For this review, take the finished solid that the model builds, in its own axes (mm). A direction names the side the tool comes from. Coordinates: 2 decimals unless noted, no trailing zeros. Write each loop counter-clockwise with the first axis right and the second up, starting at its lowest first coordinate (ties: lowest second). Pieces come first, ordered by that corner, then holes. Notation, with made-up numbers: (-32, -35) - (8, -35) arc R30 ccw to (8, -4) - close; hole circle Ø1 at (28.25, 20.5). An arc over 180 degrees is marked (long way). Write each question's results on one line, items separated by ' | '.
from build123d import *

# Parameters (mm, degrees)
F0_R     = 12.7
F1_DEPTH = 73.66
F2_R     = 5.1125641025
F3_DEPTH = 73.661
F3_TAPER = -2.9356734464
F4_R     = 12.7
F5_DEPTH = 15.24
F8_D     = 20.447
F8_DEPTH = 19.7358
F8_TIP   = 6.1428985386


with BuildPart() as f1:
    # F0 (on Top) → F1 (new body)
    with BuildSketch(Plane.XY):
        Circle(F0_R)
    extrude(amount=F1_DEPTH)

    # F2 (on Top) → F3 (cut, through all)
    with BuildSketch(Plane.XY):
        Circle(F2_R)
    extrude(amount=F3_DEPTH, taper=F3_TAPER, mode=Mode.SUBTRACT)

    # F4 (on face) → F5 (join)
    with BuildSketch(Plane.XY.offset(73.66)):
        Circle(F4_R)
    extrude(amount=F5_DEPTH)

    # F8
    with Locations(Plane.XY.offset(88.9)):
        with Locations((0, 0)):
            Hole(F8_D / 2, depth=F8_DEPTH)
            with Locations((0, 0, -(F8_DEPTH + F8_TIP / 2))):  # 118° drill point
                Cone(0, F8_D / 2, F8_TIP, mode=Mode.SUBTRACT)


solid = f1.part
Q1. Take a section at A-A on x = 0. State the section outline as (y, z) points, plus the area to 3 significant figures.
Results found:
outline: (-12.7, 0) - (-5.11, 0) - (-8.61, 68.19) - (-10.22, 69.16) - (-10.22, 88.9) - (-12.7, 88.9) - close; (5.11, 0) - (12.7, 0) - (12.7, 88.9) - (10.22, 88.9) - (10.22, 69.16) - (8.61, 68.19) - close | area: 900 mm2
Q2. Take a section at C-C on x = -11. State the section outline as (y, z) points.
Results found:
outline: (-6.35, 0) - (6.35, 0) - (6.35, 88.9) - (-6.35, 88.9) - close
Q3. Mouldability with a two-part tool opening along X and no side actions: class faces 1 (the face through (-2.75, -12.4, 43.83)), 2 (the face through (6.568, 2.068, 34.575)), 3 (the face through (5.5, 0.2, 0)) as pulls with the +X half, pulls with the -X half, needs draft (parallel to the pull), parting line crosses it, or undercut.
Results found:
face 1: parting line crosses it | face 2: undercut | face 3: needs draft
Q4. Wall thickness on line 1 along Y through (x, z) = (0, 84.75); line 2 along Y through (x, z) = (-4.25, 11.5); line 3 along X through (y, z) = (9, 74): over which ranges is each line inside the solid? List them lowest first. Write a range as from..to.
Results found:
line 1: -12.7..-10.22, 10.22..12.7 | line 2: -11.97..-3.8, 3.8..11.97 | line 3: -8.96..-4.85, 4.85..8.96
Q5. For pin 1 (6 mm diameter, centred on y = 8, z = 32, fed in from +X); pin 2 (1.5 mm diameter, centred on x = 6, z = 15, fed in from +Y), all flat-tipped, find the tip position at first contact; note any pin that passes through.
Results found:
pin 1: x = 11.67 | pin 2: y = 11.56
Q6. For faces 4 (the face through (-9, 6, 88.9)), 5 (the face through (8.113, -6.221, 78.894)), list the 3-axis set-ups (+Z, -Z, +X, -X, +Y, -Y) from which the entire face can be reached by the end or side of a thin tool; tool diameter is ignored.
Results found:
face 4: +Z, +X, -X, +Y, -Y | face 5: +Z
Q7. Take a section at B-B on z = 81.5. State the section outline as (x, y) points, plus the area to 3 significant figures.
Results found:
outline: circle Ø25.4 at (0, 0); hole circle Ø20.45 at (0, 0) | area: 178 mm2
Q8. Take a section at D-D on z = 51. State the section outline as (x, y) points, plus the area to 3 significant figures.
Results found:
outline: circle Ø25.4 at (0, 0); hole circle Ø15.46 at (0, 0) | area: 319 mm2
